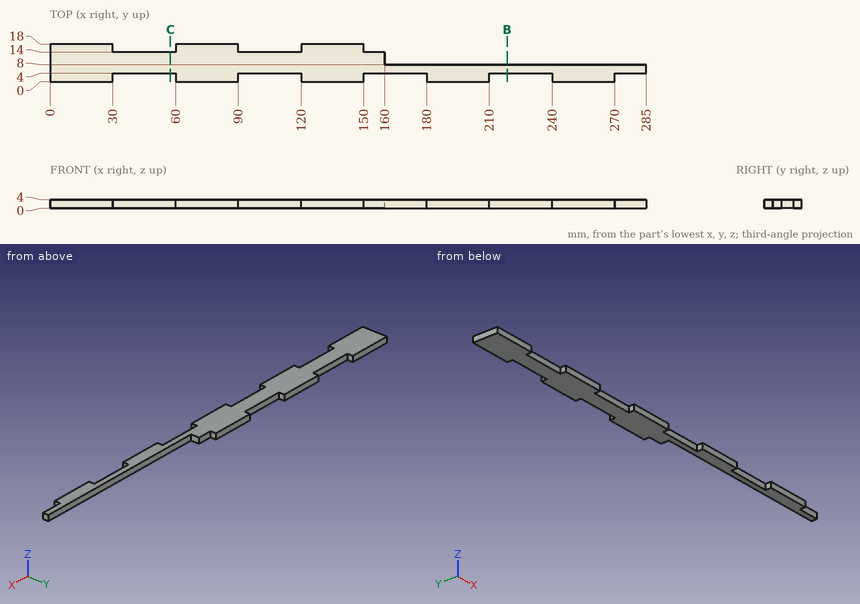
Part print with two shaded views. Sizes in mm from the minimum x, y, z corner. Give positions to 0.01 mm unless a question says otherwise; leave off trailing zeros. Order: outer loops, then holes, each group sorted by start corner. A loop starts at its lowest first (then second) coordinate and runs counter-clockwise, first axis right, second up.
(1) Flat gauge pins, fed straight in: pin 1 (2 mm diameter, centred on y = 16, z = 2.5, fed in from -X); pin 2 (1.2 mm diameter, centred on y = 12, z = 2, fed in from +X); pin 3 (2 mm diameter, centred on y = 15.5, z = 2.5, fed in from +X); pin 4 (2 mm diameter, centred on x = 280, z = 1.5, fed in from -Y). Where does each tip first touch, or does it go through?
(2) Drill centre lines: L1, parallel to X at y = 3.5, z = 3.05; L2, parallel to X at y = 16, z = 2.25; L3, parallel to X at y = 11.75, z = 1.7. Where is each one in solid material? Low to high.
(3) Saw through at C-C, the plane x = 57.5. Give the cut face in (y, z), then the cut area to 3 significant figures.
(4) Saw through at B-B, the plane x = 218.5. Give the cut face in (y, z).
Results found:
1. pin 1: stops at x = 0
1. pin 2: stops at x = 160
1. pin 3: stops at x = 150
1. pin 4: stops at y = 4
2. L1: x = 0 to 30, 60 to 90, 120 to 150, 180 to 210, 240 to 270
2. L2: x = 0 to 30, 60 to 90, 120 to 150
2. L3: x = 0 to 160
3. outline: (4, 0) - (14, 0) - (14, 4) - (4, 4) - close
3. area: 40.0 mm2
4. outline: (4, 0) - (8, 0) - (8, 4) - (4, 4) - close
